The drawing under review shows one solid part. Ordinate dimensions are in mm from its lowest x, y, z. Coordinates: 2 decimals unless noted, no trailing zeros. Write each loop counter-clockwise with the first axis right and the second up, starting at its lowest first coordinate (ties: lowest second). Pieces come first, ordered by that corner, then holes.
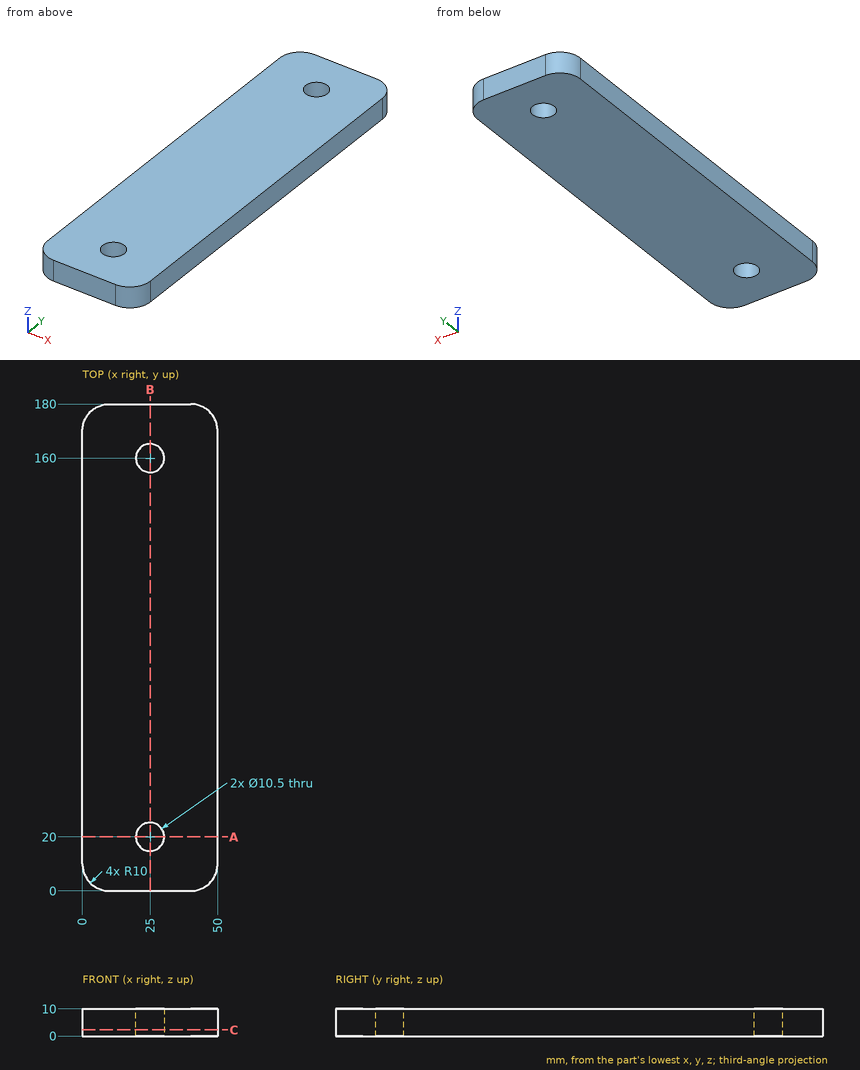
Q1. Clearance check with a flat-ended pin moving along its axis: pin 1 Ø12 at (x, y) = (25, 20) entering from -Z. State where the tip first meets the part, or that it passes through.
Ans:
pin 1: stops at z = 0
Q2. Add section C-C (z = 2.25). State the section outline as (x, y) points, then the cut area to 3 significant figures.
Ans:
outline: (0, 10) arc R10 ccw to (10, 0) - (40, 0) arc R10 ccw to (50, 10) - (50, 170) arc R10 ccw to (40, 180) - (10, 180) arc R10 ccw to (0, 170) - close; hole circle Ø10.5 at (25, 20); hole circle Ø10.5 at (25, 160)
area: 8,740 mm2
Q3. For probe 1 along Y at (x, z) = (25, 3); probe 2 along X at (y, z) = (160, 5.75); probe 3 along X at (y, z) = (158, 9), list the stretches that pass through material, from the lowest coordinate up.
Ans:
probe 1: y = 0 to 14.75, 25.25 to 154.75, 165.25 to 180
probe 2: x = 0 to 19.75, 30.25 to 50
probe 3: x = 0 to 20.15, 29.85 to 50
Q4. Add section A-A (y = 20). State the section outline as (x, z) points.
Ans:
outline: (0, 0) - (19.75, 0) - (19.75, 10) - (0, 10) - close; (30.25, 0) - (50, 0) - (50, 10) - (30.25, 10) - close
Q5. Add section B-B (x = 25). State the section outline as (y, z) points, then the cut area to 3 significant figures.
Ans:
outline: (0, 0) - (14.75, 0) - (14.75, 10) - (0, 10) - close; (25.25, 0) - (154.75, 0) - (154.75, 10) - (25.25, 10) - close; (165.25, 0) - (180, 0) - (180, 10) - (165.25, 10) - close
area: 1,590 mm2
